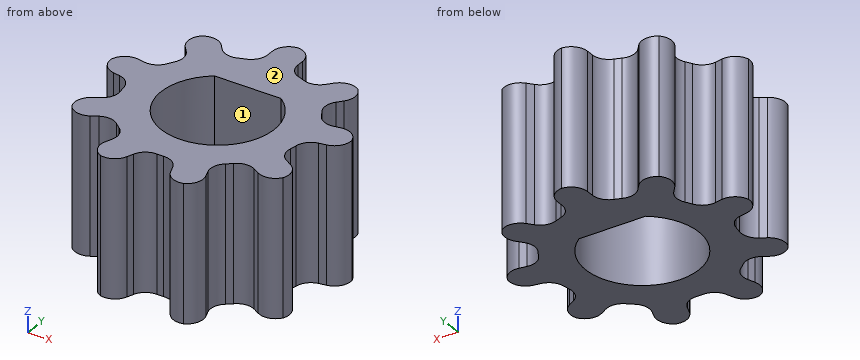
```python
from build123d import *

# Parameters (mm, degrees)
SKETCH1_R                = 2.389889751
SKETCH1_R_2              = 1.55
BOSS_EXTRUDE1_DEPTH      = 3.75
SKETCH2_W                = 0.83
SKETCH2_H                = 1
BOSS_EXTRUDE2_DEPTH      = 3.75
FILLET1_R                = 0.45
CIRPATTERN1_COUNT        = 9
FILLET1_OF_CIRPATTERN1_R = 0.45
SKETCH3_W                = 1.833030278
SKETCH3_H                = 0.3
BOSS_EXTRUDE3_DEPTH      = 3.75


with BuildPart() as part:
    # Sketch1 → Boss-Extrude1 (new body)
    with BuildSketch(Plane.XY):
        Circle(SKETCH1_R)
        Circle(SKETCH1_R_2, mode=Mode.SUBTRACT)
    extrude(amount=BOSS_EXTRUDE1_DEPTH)

    # Sketch2 → Boss-Extrude2 (add)
    with BuildSketch(Plane.XY.offset(3.75)):
        with Locations((0, 2.853581955)):
            Rectangle(SKETCH2_W, SKETCH2_H)
    boss_extrude2 = extrude(amount=-BOSS_EXTRUDE2_DEPTH)

    # Fillet1
    # the kernel refuses this fillet: 0.45 mm, written as the material it adds along each edge
    with BuildSketch(Plane(origin=(-0.415, 2.353581955, 3.75), x_dir=(-0.970855819199755, -0.2396643034036823, 0), z_dir=(0, 0, -1))) as fillet1_piece_1:
        with BuildLine():
            CenterArc((0.352674994, 0.448975623), FILLET1_R, 193.866728132, 72.266543736)
            Line((-0.084210125, 0.341126687), (0, 0))
            ThreePointArc((0, 0), (0.161164415, 0.005440327), (0.32232883, 0))
        make_face()
    extrude(amount=3.75)
    with BuildSketch(Plane(origin=(0.415, 2.353581955, 3.75), x_dir=(0.9708558191997549, -0.2396643034036833, 0), z_dir=(0, 0, -1))) as fillet1_piece_2:
        with BuildLine():
            CenterArc((0.352674994, -0.448975623), FILLET1_R, 93.866728132, 72.266543736)
            Line((-0.084210125, -0.341126687), (0, 0))
            ThreePointArc((0, 0), (0.161164415, -0.005440327), (0.32232883, 0))
        make_face()
    extrude(amount=3.75)
    # the kernel refuses this fillet: 0.45 mm, written as the material it takes off along each edge
    with BuildSketch(Plane(origin=(-0.415, 3.353581955, 4.875), x_dir=(1, 0, 0), z_dir=(0, 0, -1)), Plane(origin=(0.415, 3.353581955, 4.875), x_dir=(0, -1, 0), z_dir=(0, 0, -1))) as fillet1_2_piece_1:
        with BuildLine():
            CenterArc((FILLET1_R, FILLET1_R), FILLET1_R, 180, 90)
            Line((0, FILLET1_R), (0, 0))
            Line((0, 0), (FILLET1_R, 0))
        make_face()
    extrude(amount=6, mode=Mode.SUBTRACT)

    # CirPattern1: Boss-Extrude2 ×9 about axis
    cirpattern1_axis = Axis((0, 0, 0), (0, 0, 1))
    for i in range(1, CIRPATTERN1_COUNT):
        add(boss_extrude2.rotate(cirpattern1_axis, i * 360 / CIRPATTERN1_COUNT))

    # Fillet1 of CirPattern1
    # the kernel refuses this fillet: 0.45 mm, written as the material it adds along each edge
    with BuildSketch(Plane(origin=(-1.830761763, 1.53619152, 3.75), x_dir=(-0.5896654606556537, -0.8076475992100489, 0), z_dir=(0, 0, -1)), Plane(origin=(-2.389889751, 0, 3.75), x_dir=(0.06743592033084408, -0.9977236073428011, 0), z_dir=(0, 0, -1)), Plane(origin=(-1.830761763, -1.53619152, 3.75), x_dir=(0.6929832847277674, -0.7209536511370993, 0), z_dir=(0, 0, -1)), Plane(origin=(-0.415, -2.353581955, 3.75), x_dir=(0.994276068549242, -0.10684146905702349, 0), z_dir=(0, 0, -1)), Plane(origin=(1.194944875, -2.069705236, 3.75), x_dir=(0.8303360297488931, 0.5572630238054965, 0), z_dir=(0, 0, -1)), Plane(origin=(2.245761763, -0.817390435, 3.75), x_dir=(0.2778725344719876, 0.960617954540781, 0), z_dir=(0, 0, -1)), Plane(origin=(2.245761763, 0.817390435, 3.75), x_dir=(-0.4046106078935896, 0.9144890682670732, 0), z_dir=(0, 0, -1)), Plane(origin=(1.194944875, 2.069705236, 3.75), x_dir=(-0.8977719500797382, 0.44046058353730577, 0), z_dir=(0, 0, -1))) as fillet1_of_cirpattern1_piece_1:
        with BuildLine():
            CenterArc((0.352674994, 0.448975623), FILLET1_OF_CIRPATTERN1_R, 193.866728132, 72.266543736)
            Line((-0.084210125, 0.341126687), (0, 0))
            ThreePointArc((0, 0), (0.161164415, 0.005440327), (0.32232883, 0))
        make_face()
    extrude(amount=3.75)
    with BuildSketch(Plane(origin=(-1.194944875, 2.069705236, 3.75), x_dir=(-0.6427876096865393, 0.7660444431189779, 0), z_dir=(0, 0, -1)), Plane(origin=(-2.245761763, 0.817390435, 3.75), x_dir=(-0.9848077530122081, 0.17364817766693041, 0), z_dir=(0, 0, -1)), Plane(origin=(-2.245761763, -0.817390435, 3.75), x_dir=(-0.8660254037844392, -0.4999999999999993, 0), z_dir=(0, 0, -1)), Plane(origin=(-1.194944875, -2.069705236, 3.75), x_dir=(-0.34202014332566916, -0.9396926207859083, 0), z_dir=(0, 0, -1)), Plane(origin=(0.415, -2.353581955, 3.75), x_dir=(0.3420201433256687, -0.9396926207859083, 0), z_dir=(0, 0, -1)), Plane(origin=(1.830761763, -1.53619152, 3.75), x_dir=(0.8660254037844389, -0.49999999999999944, 0), z_dir=(0, 0, -1)), Plane(origin=(2.389889751, 0, 3.75), x_dir=(0.984807753012208, 0.1736481776669301, 0), z_dir=(0, 0, -1))) as fillet1_of_cirpattern1_piece_2:
        with BuildLine():
            CenterArc((0.35136699, 0.45), FILLET1_OF_CIRPATTERN1_R, 197.733456264, 72.266543736)
            ThreePointArc((-0.077250714, 0.31293482), (-0.033343584, 0.157771262), (0, 0))
            Line((0, 0), (0.35136699, 0))
        make_face()
    extrude(amount=3.75)
    with BuildSketch(Plane(origin=(1.830761763, 1.53619152, 3.75), x_dir=(0.5896654606556527, -0.8076475992100495, 0), z_dir=(0, 0, -1))) as fillet1_of_cirpattern1_piece_3:
        with BuildLine():
            CenterArc((0.352674994, -0.448975623), FILLET1_OF_CIRPATTERN1_R, 93.866728132, 72.266543736)
            Line((-0.084210125, -0.341126687), (0, 0))
            ThreePointArc((0, 0), (0.161164415, -0.005440327), (0.32232883, 0))
        make_face()
    extrude(amount=3.75)
    # the kernel refuses this fillet: 0.45 mm, written as the material it takes off along each edge
    with BuildSketch(Plane(origin=(-2.473549373, 2.302235963, 4.875), x_dir=(0.7660444431189787, 0.6427876096865386, 0), z_dir=(0, 0, -1)), Plane(origin=(-1.837732485, 2.835749679, 4.875), x_dir=(0.6427876096865393, -0.766044443118978, 0), z_dir=(0, 0, -1)), Plane(origin=(-3.374697504, 0.173648178, 4.875), x_dir=(0.17364817766693086, 0.984807753012208, 0), z_dir=(0, 0, -1)), Plane(origin=(-3.230569516, 0.991038613, 4.875), x_dir=(0.9848077530122081, -0.17364817766693022, 0), z_dir=(0, 0, -1)), Plane(origin=(-2.696787167, -2.03619152, 4.875), x_dir=(-0.5000000000000001, 0.8660254037844386, 0), z_dir=(0, 0, -1)), Plane(origin=(-3.111787167, -1.317390435, 4.875), x_dir=(0.8660254037844386, 0.5000000000000001, 0), z_dir=(0, 0, -1)), Plane(origin=(-0.757020143, -3.293274576, 4.875), x_dir=(-0.9396926207859084, 0.34202014332566855, 0), z_dir=(0, 0, -1)), Plane(origin=(-1.536965019, -3.009397857, 4.875), x_dir=(0.3420201433256694, 0.9396926207859081, 0), z_dir=(0, 0, -1)), Plane(origin=(1.536965019, -3.009397857, 4.875), x_dir=(-0.9396926207859084, -0.34202014332566855, 0), z_dir=(0, 0, -1)), Plane(origin=(0.757020143, -3.293274576, 4.875), x_dir=(-0.3420201433256689, 0.9396926207859084, 0), z_dir=(0, 0, -1)), Plane(origin=(3.111787167, -1.317390435, 4.875), x_dir=(-0.5000000000000004, -0.8660254037844384, 0), z_dir=(0, 0, -1)), Plane(origin=(2.696787167, -2.03619152, 4.875), x_dir=(-0.8660254037844384, 0.5000000000000004, 0), z_dir=(0, 0, -1)), Plane(origin=(3.230569516, 0.991038613, 4.875), x_dir=(0.17364817766692991, -0.9848077530122081, 0), z_dir=(0, 0, -1)), Plane(origin=(3.374697504, 0.173648178, 4.875), x_dir=(-0.9848077530122081, -0.17364817766692986, 0), z_dir=(0, 0, -1)), Plane(origin=(1.837732485, 2.835749679, 4.875), x_dir=(0.766044443118978, -0.6427876096865394, 0), z_dir=(0, 0, -1)), Plane(origin=(2.473549373, 2.302235963, 4.875), x_dir=(-0.6427876096865394, -0.766044443118978, 0), z_dir=(0, 0, -1))) as fillet1_of_cirpattern1_2_piece_1:
        with BuildLine():
            CenterArc((FILLET1_OF_CIRPATTERN1_R, FILLET1_OF_CIRPATTERN1_R), FILLET1_OF_CIRPATTERN1_R, 180, 90)
            Line((0, FILLET1_OF_CIRPATTERN1_R), (0, 0))
            Line((0, 0), (FILLET1_OF_CIRPATTERN1_R, 0))
        make_face()
    extrude(amount=6, mode=Mode.SUBTRACT)

    # Sketch3 → Boss-Extrude3 (add)
    with BuildSketch(Plane(origin=(0, 0, 0), x_dir=(-1, 0, 0), z_dir=(0, 0, -1))):
        with Locations((0, 1.4)):
            Rectangle(SKETCH3_W, SKETCH3_H)
    extrude(amount=-BOSS_EXTRUDE3_DEPTH)


solid = part.part
```
Can you work these out from the model? Positions are in its coordinate system, mm. Face numbers are marked on the shaded views. Round coordinates to 2 decimals unless told otherwise and drop trailing zeros. Order: outer loops, then holes, each group sorted by start corner. A loop starts at its lowest first (then second) coordinate and runs counter-clockwise, first axis right, second up.
(1) If we section it at A-A (y = 3.25): Please give me the cut outline in (x, z).
Results are:
outline: (-0.25, 0) - (0.25, 0) - (0.25, 3.75) - (-0.25, 3.75) - close
(2) We'd pull the mould along Y, two halves only. Please class the marked faces 1 and 2: +Y half, -Y half, draft (parallel to the pull), parting line (faces both ways), or undercut.
Results are:
face 1: undercut
face 2: draft
(3) If I drill on L1, parallel to X at y = -2.25, z = 3.1; L2, parallel to X at y = 0, z = 2.65; L3, parallel to Y at x = -2.5, z = 0.75, over which ranges is the centre line in solid material (lowest first)?
Results are:
L1: x = -1.29 to 1.29
L2: x = -2.58 to -1.55, 1.55 to 2.58
L3: y = -1.87 to -0.96, -0.06 to 0.87
